```python
from build123d import *

# Parameters (mm, degrees)
SKETCH1_W               = 279.4
SKETCH1_H               = 76.2
BOSS_EXTRUDE1_DEPTH     = 3
SKETCH3_W               = 3
SKETCH3_H               = 7.8
CUT_EXTRUDE1_DEPTH      = 145.833352512
LPATTERN1_COUNT         = 4
LPATTERN1_PITCH         = 22.8
MIRROR1_COPY_1_SKETCH_W = 3
MIRROR1_COPY_1_SKETCH_H = 7.8
MIRROR1_COPY_1_DEPTH    = 145.833352512
MIRROR1_COPY_2_SKETCH_W = 3
MIRROR1_COPY_2_SKETCH_H = 7.8
MIRROR1_COPY_2_DEPTH    = 145.833352512
MIRROR1_COPY_3_SKETCH_W = 3
MIRROR1_COPY_3_SKETCH_H = 7.8
MIRROR1_COPY_3_DEPTH    = 145.833352512
SKETCH5_W               = 3
SKETCH5_H               = 15
CUT_EXTRUDE3_DEPTH      = 10
SKETCH9_W               = 3
SKETCH9_H               = 7.8
BOSS_EXTRUDE2_DEPTH     = 3
LPATTERN4_COUNT         = 12
LPATTERN4_PITCH         = 22.8
LPATTERN5_COUNT         = 2
LPATTERN5_PITCH         = 22.8
MIRROR2_COPY_1_SKETCH_W = 3
MIRROR2_COPY_1_SKETCH_H = 15
MIRROR2_COPY_1_DEPTH    = 10


with BuildPart() as part:
    # Sketch1 → Boss-Extrude1 (new body)
    with BuildSketch(Plane(origin=(0, 0, 0), x_dir=(0, 0, -1), z_dir=(1, 0, 0))):
        Rectangle(SKETCH1_W, SKETCH1_H)
    extrude(amount=-BOSS_EXTRUDE1_DEPTH)

    # Sketch3 → Cut-Extrude1 (cut, through all)
    with BuildSketch(Plane.ZY.offset(3)):
        with Locations((-138.2, 34.2)):
            Rectangle(SKETCH3_W, SKETCH3_H)
    cut_extrude1 = extrude(amount=-CUT_EXTRUDE1_DEPTH, mode=Mode.SUBTRACT)

    # LPattern1: Cut-Extrude1 ×4
    with Locations(*[(0, -i * LPATTERN1_PITCH, 0) for i in range(1, LPATTERN1_COUNT)]):
        add(cut_extrude1, mode=Mode.SUBTRACT)

    # Mirror1: Cut-Extrude1 across plane
    add(cut_extrude1.mirror(Plane.XY), mode=Mode.SUBTRACT)

    # Mirror1 copy 1 sketch → Mirror1 copy 1 (cut, through all)
    with BuildSketch(Plane(origin=(-3, -22.8, 0), x_dir=(0, 0, -1), z_dir=(-1, 0, 0))):
        with Locations((-138.2, -34.2)):
            Rectangle(MIRROR1_COPY_1_SKETCH_W, MIRROR1_COPY_1_SKETCH_H)
    extrude(amount=-MIRROR1_COPY_1_DEPTH, mode=Mode.SUBTRACT)

    # Mirror1 copy 2 sketch → Mirror1 copy 2 (cut, through all)
    with BuildSketch(Plane(origin=(-3, -45.6, 0), x_dir=(0, 0, -1), z_dir=(-1, 0, 0))):
        with Locations((-138.2, -34.2)):
            Rectangle(MIRROR1_COPY_2_SKETCH_W, MIRROR1_COPY_2_SKETCH_H)
    extrude(amount=-MIRROR1_COPY_2_DEPTH, mode=Mode.SUBTRACT)

    # Mirror1 copy 3 sketch → Mirror1 copy 3 (cut, through all)
    with BuildSketch(Plane(origin=(-3, -68.4, 0), x_dir=(0, 0, -1), z_dir=(-1, 0, 0))):
        with Locations((-138.2, -34.2)):
            Rectangle(MIRROR1_COPY_3_SKETCH_W, MIRROR1_COPY_3_SKETCH_H)
    extrude(amount=-MIRROR1_COPY_3_DEPTH, mode=Mode.SUBTRACT)

    # Sketch5 → Cut-Extrude3 (cut)
    with BuildSketch(Plane.ZY.offset(3)):
        with Locations((-21.5, 22.8)):
            Rectangle(SKETCH5_W, SKETCH5_H)
    cut_extrude3 = extrude(amount=-CUT_EXTRUDE3_DEPTH, mode=Mode.SUBTRACT)

    # Sketch9 → Boss-Extrude2 (add)
    with BuildSketch(Plane(origin=(0, 38.1, 0), x_dir=(1, 0, 0), z_dir=(0, 1, 0))):
        with Locations((-1.5, 125.4)):
            Rectangle(SKETCH9_W, SKETCH9_H)
    boss_extrude2 = extrude(amount=BOSS_EXTRUDE2_DEPTH)

    # LPattern4: Boss-Extrude2 ×12
    with Locations(*[(0, 0, i * LPATTERN4_PITCH) for i in range(1, LPATTERN4_COUNT)]):
        add(boss_extrude2)

    # LPattern5: Cut-Extrude3 ×2
    with Locations(*[(0, -i * LPATTERN5_PITCH, 0) for i in range(1, LPATTERN5_COUNT)]):
        add(cut_extrude3, mode=Mode.SUBTRACT)

    # Mirror2: Cut-Extrude3 across plane
    add(cut_extrude3.mirror(Plane.XY), mode=Mode.SUBTRACT)

    # Mirror2 copy 1 sketch → Mirror2 copy 1 (cut)
    with BuildSketch(Plane(origin=(-3, -22.8, 0), x_dir=(0, 0, -1), z_dir=(-1, 0, 0))):
        with Locations((-21.5, -22.8)):
            Rectangle(MIRROR2_COPY_1_SKETCH_W, MIRROR2_COPY_1_SKETCH_H)
    extrude(amount=-MIRROR2_COPY_1_DEPTH, mode=Mode.SUBTRACT)


solid = part.part
```
Source: CAD feature listing. Evaluate the final solid. Frame: model axes, mm. Round coordinates to 2 decimals unless told otherwise and drop trailing zeros. Write each loop counter-clockwise with the first axis right and the second up, starting at its lowest first coordinate (ties: lowest second). Pieces come first, ordered by that corner, then holes. Notation, with made-up numbers: M -22.75,35.5 L 3.25,35.5 A18 ccw 3.25,39.5 Z; hole C 87.25,67.5 d9. An arc over 180 degrees is marked long. Use CSV: the item, a comma, the result in double quotes. Start each with the question number.
Q1. Cut plane A-A on y = 23. Output: boundary loops of the cut face in (x, z).
Q2. Cut plane B-B on x = -0.6. Count the separate pieces of the cut face and the enclosed holes in it, plus the area to 3 significant figures.
Q3. Cut plane D-D on y = 10. Output: boundary loops of the cut face in (x, z).
Q4. Line query: line 1 (Y direction, x = -1.9, z = -22); line 2 (Z direction, x = -2.15, y = -0.5); line 3 (Z direction, x = -1.9, y = 32). Output: solid intervals per line, ascending. Write a range as from..to.
Q5. First-contact query: P1, Ø1.5, axis at x = -1.5, y = 40, coming from the +Z side; P2, Ø0.9, axis at x = -1.5, z = 138.5, coming from the -Y side; P3, Ø0.9, axis at x = -1, y = -11, coming from the -Z side. Flat tips, straight axial feed; report the tip coordinate or a pass-through.
Q6. Cut plane C-C on z = -26. Output: boundary loops of the cut face in (x, y).
Results found:
1,outline,"M -3,-139.7 L 0,-139.7 L 0,-23 L -3,-23 Z; M -3,-20 L 0,-20 L 0,20 L -3,20 Z; M -3,23 L 0,23 L 0,139.7 L -3,139.7 Z"
2,separate pieces,"1"
2,enclosed holes,"4"
2,area,"21,200 mm^2"
3,outline,"M -3,-136.7 L 0,-136.7 L 0,136.7 L -3,136.7 Z"
4,line 1,"-38.1..-7.5, 7.5..15.3, 30.3..38.1"
4,line 2,"-139.7..-23, -20..20, 23..139.7"
4,line 3,"-136.7..136.7"
5,P1,"z = 129.3"
5,P2,"y = -30.3"
5,P3,"z = -136.7"
6,outline,"M -3,-38.1 L 0,-38.1 L 0,38.1 L -3,38.1 Z"
